```python
from build123d import *

# Parameters (mm, degrees)
F1_R     = 31.75
F1_R_2   = 29.36875
F2_DEPTH = 58.42
F0_R     = 29.36875
F4_DEPTH = 2.54
F5_R     = 3.175
F6_DEPTH = 58.421


with BuildPart() as f2:
    # F1 (on face) → F2 (new body)
    with BuildSketch(Plane.XY):
        Circle(F1_R)
        Circle(F1_R_2, mode=Mode.SUBTRACT)
    extrude(amount=F2_DEPTH)

    # F0 (on Top) → F4 (join)
    with BuildSketch(Plane.XY):
        Circle(F0_R)
    extrude(amount=F4_DEPTH)

    # F5 (on face) → F6 (cut, through all)
    with BuildSketch(Plane.XY):
        Circle(F5_R)
    extrude(amount=F6_DEPTH, mode=Mode.SUBTRACT)


solid = f2.part
```
Can you work these out from the model? Positions are in its coordinate system, mm. A direction names the side the tool comes from. Coordinates: 2 decimals unless noted, no trailing zeros. Order: outer loops, then holes, each group sorted by start corner. A loop starts at its lowest first (then second) coordinate and runs counter-clockwise, first axis right, second up.
1. If we section it at B-B (y = 2): Please give me the cut outline in (x, z).
2. I'm going to push flat-ended pins straight in: pin 1 (2 mm diameter, centred on y = -15.5, z = 39.5, fed in from +X); pin 2 (5 mm diameter, centred on x = -3.5, y = 9.5, fed in from +Z); pin 3 (1 mm diameter, centred on x = -25.5, y = -20, fed in from +Z); pin 4 (1 mm diameter, centred on x = -8.5, z = 28.5, fed in from +Y). Where does each tip first touch, or does it pass through?
3. If we section it at D-D (y = 20.5): Please give me the cut outline in (x, z).
4. For faces 4 (the face through (7, 0, 0)), 5 (the face through (0, -6, 2.54)), which set-ups out of +Z, -Z, +X, -X, +Y, -Y let a thin tool reach every point of the face, with its end or its side?
5. If we section it at A-A (x = 0): Please give me the cut outline in (y, z) (3 decimals), then the cut area to 3 significant figures.
6. If we section it at C-C (z = 45.5): Please give me the cut outline in (x, y), then the cut area to 3 significant figures.
7. Thinking about a two-plate mould opening in Y: for faces 1 (the face through (28.1, -9.3, 58.42)), 2 (the face through (-6.883, -30.995, 28.801)), 3 (the face through (-23.306, -17.87, 30.089)), which applies, +Y half, -Y half, draft (parallel to the pull), parting line (faces both ways), or undercut?
8. I need wall thicknesses on line 1 (Y direction, x = 0, z = 0.65) (3 decimals); line 2 (Y direction, x = 0, z = 35); line 3 (Z direction, x = 17, y = -2.5). Which ranges of each line are inside material? Lowest first, please.
Entries:
1. outline: (-31.69, 0) - (-2.47, 0) - (-2.47, 2.54) - (-29.3, 2.54) - (-29.3, 58.42) - (-31.69, 58.42) - close; (2.47, 0) - (31.69, 0) - (31.69, 58.42) - (29.3, 58.42) - (29.3, 2.54) - (2.47, 2.54) - close
2. pin 1: stops at x = 28.25
2. pin 2: stops at z = 2.54
2. pin 3: passes through
2. pin 4: stops at y = 30.73
3. outline: (-24.24, 0) - (24.24, 0) - (24.24, 58.42) - (21.03, 58.42) - (21.03, 2.54) - (-21.03, 2.54) - (-21.03, 58.42) - (-24.24, 58.42) - close
4. face 4: -Z, +X, -X, +Y, -Y
4. face 5: +Z
5. outline: (-31.75, 0) - (-3.175, 0) - (-3.175, 2.54) - (-29.369, 2.54) - (-29.369, 58.42) - (-31.75, 58.42) - close; (3.175, 0) - (31.75, 0) - (31.75, 58.42) - (29.369, 58.42) - (29.369, 2.54) - (3.175, 2.54) - close
5. area: 411 mm2
6. outline: circle Ø63.5 at (0, 0); hole circle Ø58.74 at (0, 0)
6. area: 457 mm2
7. face 1: draft
7. face 2: parting line
7. face 3: undercut
8. line 1: y = -31.75 to -3.175, 3.175 to 31.75
8. line 2: y = -31.75 to -29.37, 29.37 to 31.75
8. line 3: z = 0 to 2.54
